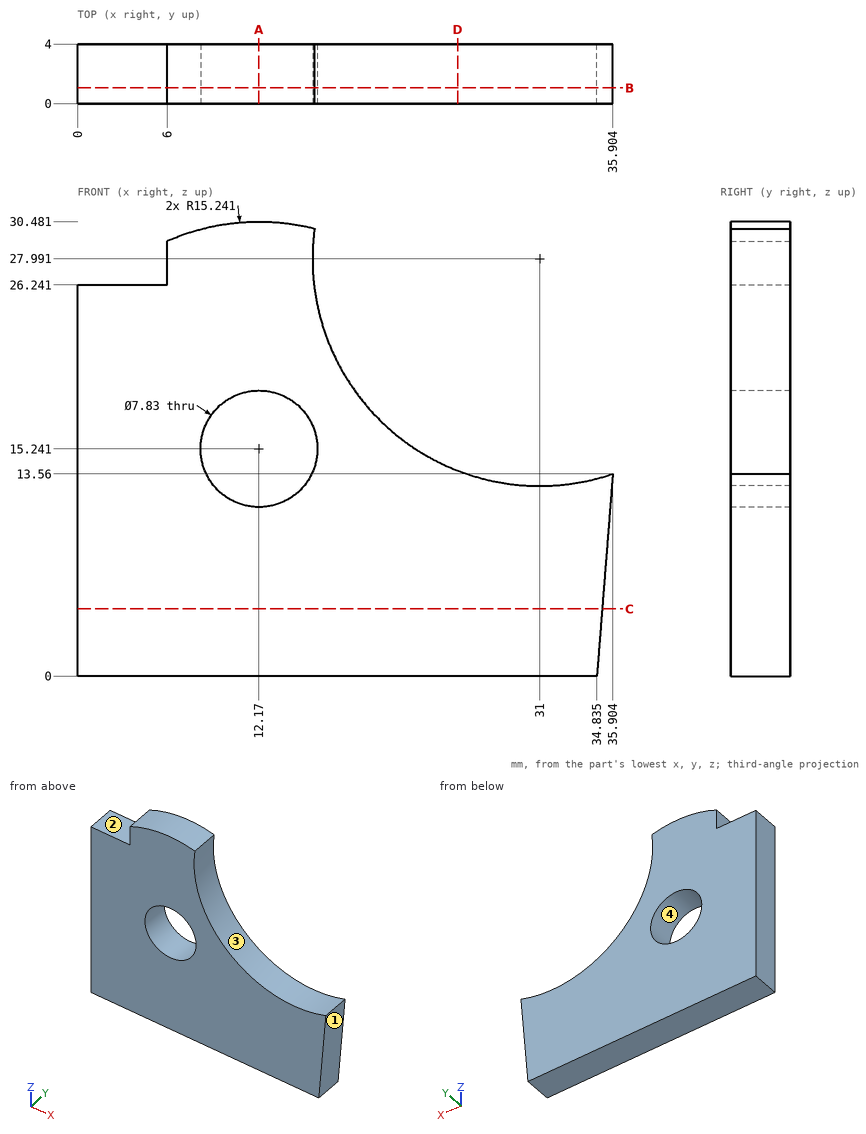
Geometry: see drawing. Coordinates: mm, zero at the bounding-box minimum. Round coordinates to 2 decimals unless told otherwise and drop trailing zeros. Write each loop counter-clockwise with the first axis right and the second up, starting at its lowest first coordinate (ties: lowest second). Pieces come first, ordered by that corner, then holes.
1) Draft query along X for the marked faces 1, 2, 3 and 4. Return one class per face: pulls with the +X half, pulls with the -X half, needs draft (parallel to the pull), parting line crosses it, or undercut.
2) Contact query for flat-ended pins moving along their axis: P1, Ø2, axis at x = 27.5, y = 1.5, coming from the +Z side; P2, Ø2, axis at x = 20.5, y = 2.5, coming from the +Z side; P3, Ø1.2, axis at x = 2.5, y = 2.5, coming from the +Z side. Output: stop coordinate, or through.
3) Cut plane A-A (x = 12.17). Return the cut outline in (y, z) (1 decimal).
4) Cut plane C-C (z = 4.5). Return the cut outline in (x, y), then the cut area to 3 significant figures.
5) Ray query, L1, parallel to X at y = 0.7, z = 28; L2, parallel to Z at x = 4, y = 2; L3, parallel to X at y = 2.95, z = 16.5 (1 decimal). Return the intervals inside material, ascending.
6) Cut plane B-B (y = 1.05). Return the cut outline in (x, z) (1 decimal).
7) Cut plane D-D (x = 25.5). Return the cut outline in (y, z), then the cut area to 3 significant figures.
Geometry says:
1. face 1: pulls with the +X half
1. face 2: needs draft
1. face 3: undercut
1. face 4: undercut
2. P1: stops at z = 13.43
2. P2: stops at z = 17.99
2. P3: stops at z = 26.24
3. outline: (0, 0) - (4, 0) - (4, 11.3) - (0, 11.3) - close; (0, 19.2) - (4, 19.2) - (4, 30.5) - (0, 30.5) - close
4. outline: (0, 0) - (35.19, 0) - (35.19, 4) - (0, 4) - close
4. area: 141 mm2
5. L1: x = 6 to 15.76
5. L2: z = 0 to 26.24
5. L3: x = 0 to 8.5, 15.9 to 21
6. outline: (0, 0) - (34.8, 0) - (35.9, 13.6) arc R15.2 cw to (15.9, 30) arc R15.2 ccw to (6, 29.2) - (6, 26.2) - (0, 26.2) - close; hole circle Ø7.8 at (12.2, 15.2)
7. outline: (0, 0) - (4, 0) - (4, 13.78) - (0, 13.78) - close
7. area: 55.1 mm2
